from build123d import *

# Parameters (mm, degrees)
SKETCH2_W                                       = 80
SKETCH2_H                                       = 36
BOSS_EXTRUDE2_DEPTH                             = 8
SKETCH3_W                                       = 71.5
SKETCH3_H                                       = 25
CUT_EXTRUDE1_DEPTH                              = 8
CSK_FOR_M3_FLAT_HEAD_MACHINE_SCREW1_D           = 3.2
CSK_FOR_M3_FLAT_HEAD_MACHINE_SCREW1_CSINK_D     = 6.3
CSK_FOR_M3_FLAT_HEAD_MACHINE_SCREW1_CSINK_ANGLE = 90
CUT_EXTRUDE2_DEPTH                              = 45.586993619
CUT_EXTRUDE2_DEPTH_BACK                         = 3.5


with BuildPart() as part:
    # Sketch2 → Boss-Extrude2 (new body)
    with BuildSketch(Plane.XY):
        Rectangle(SKETCH2_W, SKETCH2_H)
    extrude(amount=BOSS_EXTRUDE2_DEPTH)

    # Sketch3 → Cut-Extrude1 (cut)
    with BuildSketch(Plane.XY.offset(8)):
        Rectangle(SKETCH3_W, SKETCH3_H)
    extrude(amount=-CUT_EXTRUDE1_DEPTH, mode=Mode.SUBTRACT)

    # CSK for M3 Flat Head Machine Screw1 (through all)
    with Locations(Plane.XY.offset(8)):
        with Locations((-37.5, 15.5), (-37.5, -15.5), (37.5, 15.5), (37.5, -15.5)):
            CounterSinkHole(CSK_FOR_M3_FLAT_HEAD_MACHINE_SCREW1_D / 2, CSK_FOR_M3_FLAT_HEAD_MACHINE_SCREW1_CSINK_D / 2, counter_sink_angle=CSK_FOR_M3_FLAT_HEAD_MACHINE_SCREW1_CSINK_ANGLE)

    # Sketch7 → Cut-Extrude2 (cut, two sides: drawn at the far end of the back side and taken through both)
    with BuildSketch(Plane(origin=(0, 0, 0), x_dir=(-1, 0, 0), z_dir=(0, 0, -1)).offset(-CUT_EXTRUDE2_DEPTH_BACK)):
        Polygon((-35.75, -8.5), (-35.75, 8.5), (-39.75, 6.5), (-39.75, -6.5), align=None)
    extrude(amount=CUT_EXTRUDE2_DEPTH + CUT_EXTRUDE2_DEPTH_BACK, mode=Mode.SUBTRACT)


solid = part.part
Can you work these out from the model? Positions are in its coordinate system, mm. A direction names the side the tool comes from. Give positions to 0.01 mm unless a question says otherwise; leave off trailing zeros. Loops run counter-clockwise (first coordinate to the right, second up) from the corner with the lowest first, then second, coordinate; pieces in that order, holes last. Notation, with made-up numbers: (25.5, 13.25) -> (51.5, 13.25) arc R21 ccw to (51.5, 41.25) -> close; hole circle Ø11 at (-31.75, -1). An arc over 180 degrees is marked (long way). Return JSON: item names as keys, results as strings.
Q1. For pin 1 Ø3.5 at (x, y) = (37.5, -15.5) entering from -Z; pin 2 Ø2 at (x, y) = (37.5, -1.5) entering from -Z, each with a flat end and sliding along its axis, tell me the tip position at first contact or that it passes through.
Checks:
{"pin 1": "stops at z = 0", "pin 2": "stops at z = 3.5"}
Q2. I want a section at B-B, the plane x = 0.5. List the corners of the cut face in (y, z) for me.
Checks:
{"outline": "(-18, 0) -> (-12.5, 0) -> (-12.5, 8) -> (-18, 8) -> close; (12.5, 0) -> (18, 0) -> (18, 8) -> (12.5, 8) -> close"}
Q3. I want a section at A-A, the plane y = -10. List the corners of the cut face in (x, z) for me.
Checks:
{"outline": "(-40, 0) -> (-35.75, 0) -> (-35.75, 8) -> (-40, 8) -> close; (35.75, 0) -> (40, 0) -> (40, 8) -> (35.75, 8) -> close"}
Q4. We'd pull the mould along Y, two halves only. Please class faces 4 (the face through (-36.14, -14.25, 6.7)), 5 (the face through (-1, 18, 4)), 6 (the face through (37.708, -13.914, 3.18)), 7 (the face through (0, 13, 8)): released by +Y, released by -Y, zero draft, split by the parting line, or undercut.
Checks:
{"face 4": "undercut", "face 5": "released by +Y", "face 6": "undercut", "face 7": "zero draft"}
Q5. On a 3-axis mill with a long thin cutter (end or side, diameter ignored), from which of +Z, -Z, +X, -X, +Y, -Y can I reach the whole of each face in a straight line? I mean faces 1 (the face through (40, 0, 4)), 2 (the face through (37.778, -7.486, 1.774)), 3 (the face through (35.75, 0, 5)). Say none if no direction works.
Checks:
{"face 1": "+Z, -Z, +X, +Y, -Y", "face 2": "-Z", "face 3": "+Z, -Z"}
Q6. I want a section at C-C, the plane y = -15.5. List the corners of the cut face in (x, z) for me, then the cut area to 3 significant figures.
Checks:
{"outline": "(-40, 0) -> (-39.1, 0) -> (-39.1, 6.45) -> (-40, 7.35) -> close; (-35.9, 0) -> (35.9, 0) -> (35.9, 6.45) -> (34.35, 8) -> (-34.35, 8) -> (-35.9, 6.45) -> close; (39.1, 0) -> (40, 0) -> (40, 7.35) -> (39.1, 6.45) -> close", "area": "584 mm2"}
Q7. I need wall thicknesses on probe 1 along X at (y, z) = (15.5, 4.25); probe 2 along Y at (x, z) = (-37.5, 4.25); probe 3 along X at (y, z) = (4, 5.25). Which ranges of each line are inside material? Lowest first, please.
Checks:
{"probe 1": "x = -40 to -39.1, -35.9 to 35.9, 39.1 to 40", "probe 2": "y = -18 to -17.1, -13.9 to 13.9, 17.1 to 18", "probe 3": "x = -40 to -35.75, 35.75 to 40"}
Q8. I want a section at D-D, the plane x = -37.5. List the corners of the cut face in (y, z) for me, then the cut area to 3 significant figures.
Checks:
{"outline": "(-18, 0) -> (-17.1, 0) -> (-17.1, 6.45) -> (-18, 7.35) -> close; (-13.9, 0) -> (13.9, 0) -> (13.9, 6.45) -> (12.35, 8) -> (-12.35, 8) -> (-13.9, 6.45) -> close; (17.1, 0) -> (18, 0) -> (18, 7.35) -> (17.1, 6.45) -> close", "area": "232 mm2"}
